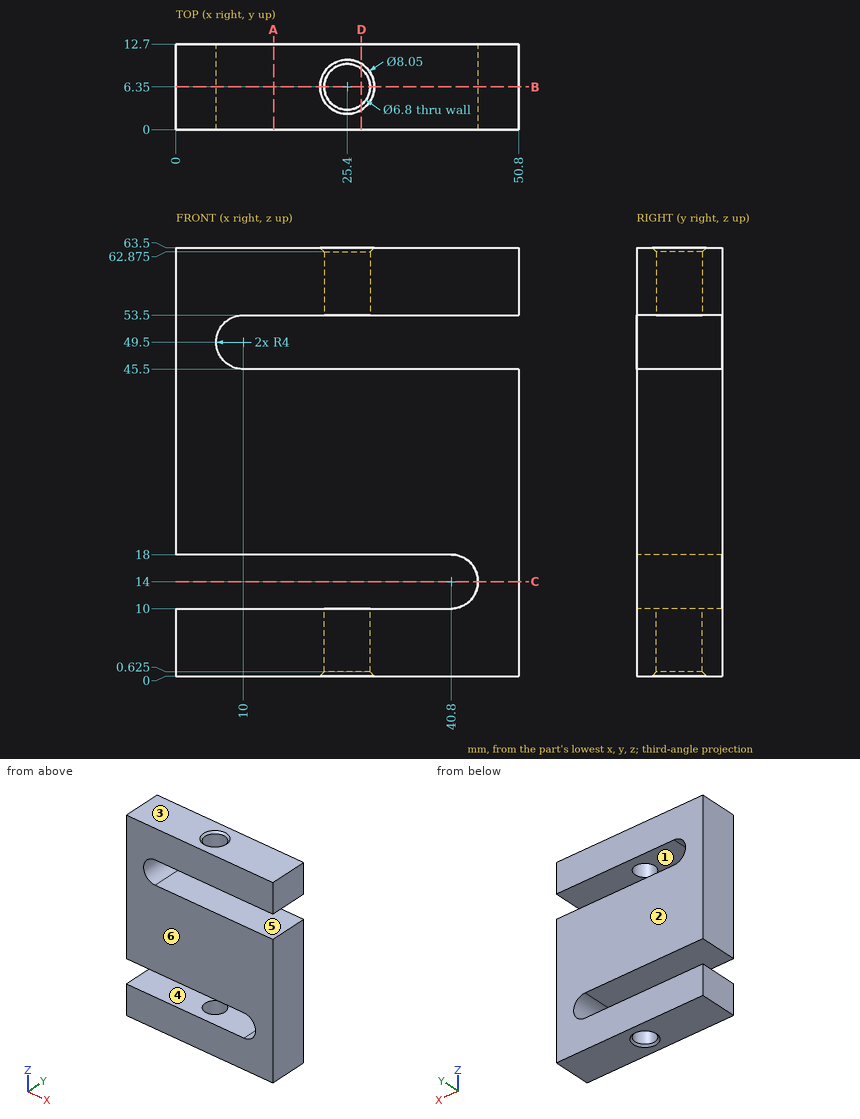
Check sheet for the drawn part. Datum: minimum x, y, z corner. Units: mm. A direction names the side the tool comes from. Coordinates: 2 decimals unless noted, no trailing zeros. Loops run counter-clockwise (first coordinate to the right, second up) from the corner with the lowest first, then second, coordinate; pieces in that order, holes last. Notation, with made-up numbers: (82, 14) -> (126, 14) arc R15 cw to (126, 28) -> close; hole circle Ø11 at (49, 49). An arc over 180 degrees is marked (long way). Answer in a Markdown table with one row per item.
1) Draft check along Z on the marked faces 1, 2 and 3. Enter one of: released by +Z, released by -Z, zero draft, split by the parting line, or undercut.
The answers:
| item | result |
|---|---|
| face 1 | undercut |
| face 2 | zero draft |
| face 3 | released by +Z |
2) Access from +Z, -Z, +X, -X, +Y, -Y to the whole of each face (thin tool, end or side, straight path). Record for the marked faces 4, 5 and 6.
The answers:
| item | result |
|---|---|
| face 4 | -X, +Y, -Y |
| face 5 | +X, +Y, -Y |
| face 6 | +Z, -Z, +X, -X, -Y |
3) Section check C-C (z = 14). Record the cut outline in (x, y), and give its area (3 significant figures).
The answers:
| item | result |
|---|---|
| outline | (44.8, 0) -> (50.8, 0) -> (50.8, 12.7) -> (44.8, 12.7) -> close |
| area | 76.2 mm2 |
4) Scan lines: line 1 along Z through (x, y) = (21, 3.25); line 2 along Z through (x, y) = (2, 5.25); line 3 along X through (y, z) = (6.35, 5). Record each from-to range of solid material in increasing order. Write a range as from..to.
The answers:
| item | result |
|---|---|
| line 1 | z = 0..10, 18..45.5, 53.5..63.5 |
| line 2 | z = 0..10, 18..63.5 |
| line 3 | x = 0..22, 28.8..50.8 |
5) Section check A-A (x = 14.5). Record the cut outline in (y, z).
The answers:
| item | result |
|---|---|
| outline | (0, 0) -> (12.7, 0) -> (12.7, 10) -> (0, 10) -> close; (0, 18) -> (12.7, 18) -> (12.7, 45.5) -> (0, 45.5) -> close; (0, 53.5) -> (12.7, 53.5) -> (12.7, 63.5) -> (0, 63.5) -> close |
6) Depth check by flat-ended pin: P1, Ø1, axis at x = 7.5, z = 56.5, coming from the -Y side; P2, Ø5, axis at y = 5.5, z = 13, coming from the -X side; P3, Ø5, axis at y = 6.5, z = 49.5, coming from the +X side; P4, Ø5.5, axis at x = 25.4, y = 6.35, coming from the -Z side. Enter the tip coordinate at first touch or a pass-through.
The answers:
| item | result |
|---|---|
| P1 | stops at y = 0 |
| P2 | stops at x = 42.74 |
| P3 | stops at x = 6.88 |
| P4 | stops at z = 18 |
7) Section check B-B (y = 6.35). Record the cut outline in (x, z) (3 decimals).
The answers:
| item | result |
|---|---|
| outline | (0, 0) -> (21.375, 0) -> (22, 0.625) -> (22, 10) -> (0, 10) -> close; (0, 18) -> (40.8, 18) arc R4 cw to (40.8, 10) -> (28.8, 10) -> (28.8, 0.625) -> (29.425, 0) -> (50.8, 0) -> (50.8, 45.5) -> (10, 45.5) arc R4 cw to (10, 53.5) -> (22, 53.5) -> (22, 62.875) -> (21.375, 63.5) -> (0, 63.5) -> close; (28.8, 53.5) -> (50.8, 53.5) -> (50.8, 63.5) -> (29.425, 63.5) -> (28.8, 62.875) -> close |
8) Section check D-D (x = 27.5). Give the number of separate pieces and of enclosed holes in the cut face, and give its area (3 significant figures).
The answers:
| item | result |
|---|---|
| separate pieces | 5 |
| enclosed holes | 0 |
| area | 495 mm2 |
